from build123d import *

# Parameters (mm, degrees)
SKETCH1_R           = 1.9
BOSS_EXTRUDE1_DEPTH = 6
SKETCH2_W           = 40
SKETCH2_H           = 5
CUT_EXTRUDE1_DEPTH  = 59.49778203


with BuildPart() as part:
    # Sketch1 → Boss-Extrude1 (new body)
    with BuildSketch(Plane.XY):
        with BuildLine():
            Line((-52.97405025, 5), (52.97405025, 5))
            ThreePointArc((52.97405025, 5), (57.97405025, 0), (52.97405025, -5))
            Line((52.97405025, -5), (-52.97405025, -5))
            ThreePointArc((-52.97405025, -5), (-57.97405025, 0), (-52.97405025, 5))
        make_face()
        with Locations((-52.97405025, 0)):
            Circle(SKETCH1_R, mode=Mode.SUBTRACT)
        with Locations((52.97405025, 0)):
            Circle(SKETCH1_R, mode=Mode.SUBTRACT)
    extrude(amount=BOSS_EXTRUDE1_DEPTH)

    # Sketch2 → Cut-Extrude1 (cut, through all)
    with BuildSketch(Plane.XY.offset(6)):
        with Locations((-25, 0)):
            Rectangle(SKETCH2_W, SKETCH2_H)
        with Locations((25, 0)):
            Rectangle(SKETCH2_W, SKETCH2_H)
    extrude(amount=-CUT_EXTRUDE1_DEPTH, mode=Mode.SUBTRACT)


solid = part.part
Source: CAD feature listing. Evaluate the final solid. Frame: model axes, mm. A direction names the side the tool comes from. Round coordinates to 2 decimals unless told otherwise and drop trailing zeros. Loops run counter-clockwise (first coordinate to the right, second up) from the corner with the lowest first, then second, coordinate; pieces in that order, holes last. Notation, with made-up numbers: M 67,14 L 76,14 A21 ccw 76,45 Z; hole C 37.25,70.25 d11. An arc over 180 degrees is marked long. Return JSON: item names as keys, results as strings. Group by question number.
1. Mould query, pull axis X, two halves, no side actions, for faces 1 (the face through (57.973, 0.11, 2.958)), 2 (the face through (45, 0, 3)), 3 (the face through (1, 0, 0)). Classes: released by +X, released by -X, zero draft, split by the parting line, or undercut.
2. Pin query (flat end, axial travel): pin 1 (1 mm diameter, centred on x = 18.5, y = -0.5, fed in from +Z); pin 2 (1.5 mm diameter, centred on y = -4, z = 2.5, fed in from +X); pin 3 (2 mm diameter, centred on y = 1.5, z = 5.5, fed in from +X). Return the tip coordinate at first contact, or that it passes through.
3. Section query A-A on y = 0. Output: boundary loops of the cut face in (x, z), and give its area (3 significant figures).
4. Reachability of faces 4 (the face through (1, 0, 6)), 5 (the face through (-45, 0, 3)) from +Z, -Z, +X, -X, +Y, -Y: full face, straight path, thin tool, end or side. Return the list, or none.
5. Section query C-C on z = 3.5. Output: boundary loops of the cut face in (x, y), and give its area (3 significant figures).
6. Section query B-B on x = 13. Output: boundary loops of the cut face in (y, z), and give its area (3 significant figures).
7. Material intervals for line 1 along X through (y, z) = (-0.25, 5.75); line 2 along Y through (x, z) = (6, 4.4); line 3 along X through (y, z) = (1, 1), sorted ascending. Write a range as from..to.
Checks:
{
 "1": {"face 1": "released by +X", "face 2": "undercut", "face 3": "zero draft"},
 "2": {"pin 1": "passes through", "pin 2": "stops at x = 56.77", "pin 3": "stops at x = 57.95"},
 "3": {"outline": "M -57.97,0 L -54.87,0 L -54.87,6 L -57.97,6 Z; M -51.07,0 L -45,0 L -45,6 L -51.07,6 Z; M -5,0 L 5,0 L 5,6 L -5,6 Z; M 45,0 L 51.07,0 L 51.07,6 L 45,6 Z; M 54.87,0 L 57.97,0 L 57.97,6 L 54.87,6 Z", "area": "170 mm²"},
 "4": {"face 4": "+Z, +X, -X, +Y, -Y", "face 5": "+Z, -Z"},
 "5": {"outline": "M -52.97,-5 L 52.97,-5 A5 ccw 52.97,5 L -52.97,5 A5 ccw Z; hole C -52.97,0 d3.8; hole M -45,-2.5 L -5,-2.5 L -5,2.5 L -45,2.5 Z; hole M 5,-2.5 L 45,-2.5 L 45,2.5 L 5,2.5 Z; hole C 52.97,0 d3.8", "area": "715 mm²"},
 "6": {"outline": "M -5,0 L -2.5,0 L -2.5,6 L -5,6 Z; M 2.5,0 L 5,0 L 5,6 L 2.5,6 Z", "area": "30.0 mm²"},
 "7": {"line 1": "x = -57.97..-54.86, -51.09..-45, -5..5, 45..51.09, 54.86..57.97", "line 2": "y = -5..-2.5, 2.5..5", "line 3": "x = -57.87..-54.59, -51.36..-45, -5..5, 45..51.36, 54.59..57.87"}
}
